Here's how the part is built. I have some questions about the finished solid (model axes, mm). A direction names the side the tool comes from. Give positions to 0.01 mm unless a question says otherwise; leave off trailing zeros. Order: outer loops, then holes, each group sorted by start corner. A loop starts at its lowest first (then second) coordinate and runs counter-clockwise, first axis right, second up. Notation, with made-up numbers: (-32.75, 33.25) -> (-22.75, 33.25) arc R16 cw to (-22.75, 44.25) -> close; hole circle Ø1 at (79, 72). An arc over 180 degrees is marked (long way). Write each question's results on one line, items separated by ' | '. Start each with the question number.
Q1. Imagine slicing it at B-B, the plane x = 64. Please give me the cut outline in (y, z), then the cut area to 3 significant figures.
Q2. Imagine slicing it at D-D, the plane y = 44. Please give me the cut outline in (x, z), then the cut area to 3 significant figures.
Q3. Imagine slicing it at C-C, the plane z = 1.5. State how many separate pieces and enclosed holes the cut face has, then the cut area to 3 significant figures.
Q4. Thinking about a two-plate mould opening in X: for faces 1 (the face through (70, 59, 1)), 2 (the face through (49.835, 6.921, 3.549)), 3 (the face through (8, 59, 7)), 4 (the face through (8.115, 55.395, 4.972)), which applies, pulls with the +X half, pulls with the -X half, needs draft (parallel to the pull), parting line crosses it, or undercut?
Q5. I need wall thicknesses on line 1 along Y through (x, z) = (35, 2.75); line 2 along Y through (x, z) = (48.5, 4); line 3 along Y through (x, z) = (26, 2). Which ranges of each line are inside material? Lowest first, please. Write a range as [from, to].
Q6. I'm going to push flat-ended pins straight in: pin 1 (8.5 mm diameter, centred on x = 64, y = 6, fed in from -Z); pin 2 (8.5 mm diameter, centred on x = 64, y = 59, fed in from +Z); pin 3 (3.5 mm diameter, centred on y = 39, z = 1.5, fed in from +X). Where does each tip first touch, or does it pass through?
Q7. Imagine slicing it at A-A, the plane z = 6. Please give me the cut outline in (x, y), then the cut area to 3 significant figures.
Q8. For faces 5 (the face through (36.372, 45.879, 1.521)), 6 (the face through (5.741, 3.083, 4.972)), 7 (the face through (69.1, 53.86, 1.48)), which set-ups out of +Z, -Z, +X, -X, +Y, -Y let a thin tool reach every point of the face, with its end or its side?
```python
from build123d import *

# Parameters (mm, degrees)
SKETCH1_R           = 2.6
BOSS_EXTRUDE1_DEPTH = 3
SKETCH2_R           = 3.5
BOSS_EXTRUDE2_DEPTH = 4
CUT_EXTRUDE1_DEPTH  = 3
SKETCH4_R           = 1.4
CUT_EXTRUDE2_DEPTH  = 96.781000204


with BuildPart() as part:
    # Sketch1 → Boss-Extrude1 (new body)
    with BuildSketch(Plane.XY):
        with BuildLine():
            ThreePointArc((0, 3), (0.878679656, 0.878679656), (3, 0))
            Line((3, 0), (67, 0))
            ThreePointArc((67, 0), (69.121320344, 0.878679656), (70, 3))
            Line((70, 3), (70, 9))
            ThreePointArc((70, 9), (69.121320344, 11.121320344), (67, 12))
            Line((67, 12), (58, 12))
            ThreePointArc((58, 12), (55.878679656, 12.878679656), (55, 15))
            Line((55, 15), (55, 50))
            ThreePointArc((55, 50), (55.878679656, 52.121320344), (58, 53))
            Line((58, 53), (67, 53))
            ThreePointArc((67, 53), (69.121320344, 53.878679656), (70, 56))
            Line((70, 56), (70, 62))
            ThreePointArc((70, 62), (69.121320344, 64.121320344), (67, 65))
            Line((67, 65), (62, 65))
            Line((62, 65), (3, 65))
            ThreePointArc((3, 65), (0.878679656, 64.121320344), (0, 62))
            Line((0, 62), (0, 3))
        make_face()
        with Locations((64, 6)):
            Circle(SKETCH1_R, mode=Mode.SUBTRACT)
        with Locations((64, 59)):
            Circle(SKETCH1_R, mode=Mode.SUBTRACT)
    extrude(amount=BOSS_EXTRUDE1_DEPTH)

    # Sketch2 → Boss-Extrude2 (add)
    with BuildSketch(Plane.XY.offset(3)):
        with Locations((6.5, 58.5)):
            Circle(SKETCH2_R)
        with Locations((48.5, 58.5)):
            Circle(SKETCH2_R)
        with Locations((6.5, 6.5)):
            Circle(SKETCH2_R)
        with Locations((48.5, 6.5)):
            Circle(SKETCH2_R)
    extrude(amount=BOSS_EXTRUDE2_DEPTH)

    # Sketch3 → Cut-Extrude1 (cut)
    with BuildSketch(Plane.XY.offset(3)):
        Polygon((10, 55), (45, 55), (27.5, 36.5), align=None)
        Polygon((50, 50), (50, 15), (31.5, 32.5), align=None)
        Polygon((45, 10), (10, 10), (27.5, 28.5), align=None)
        Polygon((5, 15), (5, 50), (23.5, 32.5), align=None)
    extrude(amount=-CUT_EXTRUDE1_DEPTH, mode=Mode.SUBTRACT)

    # Sketch4 → Cut-Extrude2 (cut, through all)
    with BuildSketch(Plane.XY.offset(7)):
        with Locations((6.5, 58.5)):
            Circle(SKETCH4_R)
        with Locations((48.5, 6.5)):
            Circle(SKETCH4_R)
        with Locations((6.5, 6.5)):
            Circle(SKETCH4_R)
        with Locations((48.5, 58.5)):
            Circle(SKETCH4_R)
    extrude(amount=-CUT_EXTRUDE2_DEPTH, mode=Mode.SUBTRACT)


solid = part.part
```
Geometry check:
1) outline: (0, 0) -> (3.4, 0) -> (3.4, 3) -> (0, 3) -> close; (8.6, 0) -> (12, 0) -> (12, 3) -> (8.6, 3) -> close; (53, 0) -> (56.4, 0) -> (56.4, 3) -> (53, 3) -> close; (61.6, 0) -> (65, 0) -> (65, 3) -> (61.6, 3) -> close | area: 40.8 mm²
2) outline: (0, 0) -> (5, 0) -> (5, 3) -> (0, 3) -> close; (11.34, 0) -> (20.41, 0) -> (20.41, 3) -> (11.34, 3) -> close; (34.59, 0) -> (43.66, 0) -> (43.66, 3) -> (34.59, 3) -> close; (50, 0) -> (55, 0) -> (55, 3) -> (50, 3) -> close | area: 84.4 mm²
3) separate pieces: 1 | enclosed holes: 10 | area: 2,570 mm²
4) face 1: pulls with the +X half | face 2: undercut | face 3: needs draft | face 4: undercut
5) line 1: [0, 10], [20.57, 29.19], [35.81, 44.43], [55, 65] | line 2: [3, 5.1], [7.9, 10], [55, 57.1], [59.9, 62] | line 3: [0, 10], [26.91, 38.09], [55, 65]
6) pin 1: z = 0 | pin 2: z = 3 | pin 3: x = 55
7) outline: circle Ø7 at (6.5, 6.5); circle Ø7 at (6.5, 58.5); circle Ø7 at (48.5, 6.5); circle Ø7 at (48.5, 58.5); hole circle Ø2.8 at (6.5, 6.5); hole circle Ø2.8 at (6.5, 58.5); hole circle Ø2.8 at (48.5, 6.5); hole circle Ø2.8 at (48.5, 58.5) | area: 129 mm²
8) face 5: +Z, -Z | face 6: +Z | face 7: +Z, -Z, +X
